Answer from the drawing. Dimensions are ordinates in mm from the lowest x, y and z of the part. Round coordinates to 2 decimals unless told otherwise and drop trailing zeros. Loops run counter-clockwise (first coordinate to the right, second up) from the corner with the lowest first, then second, coordinate; pieces in that order, holes last. Notation, with made-up numbers: M -30.75,-1 L 17.25,-1 A23 ccw 17.25,23 Z; hole C 16.25,21 d9. An arc over 180 degrees is marked long. Answer as a JSON object with one key per item and string values.
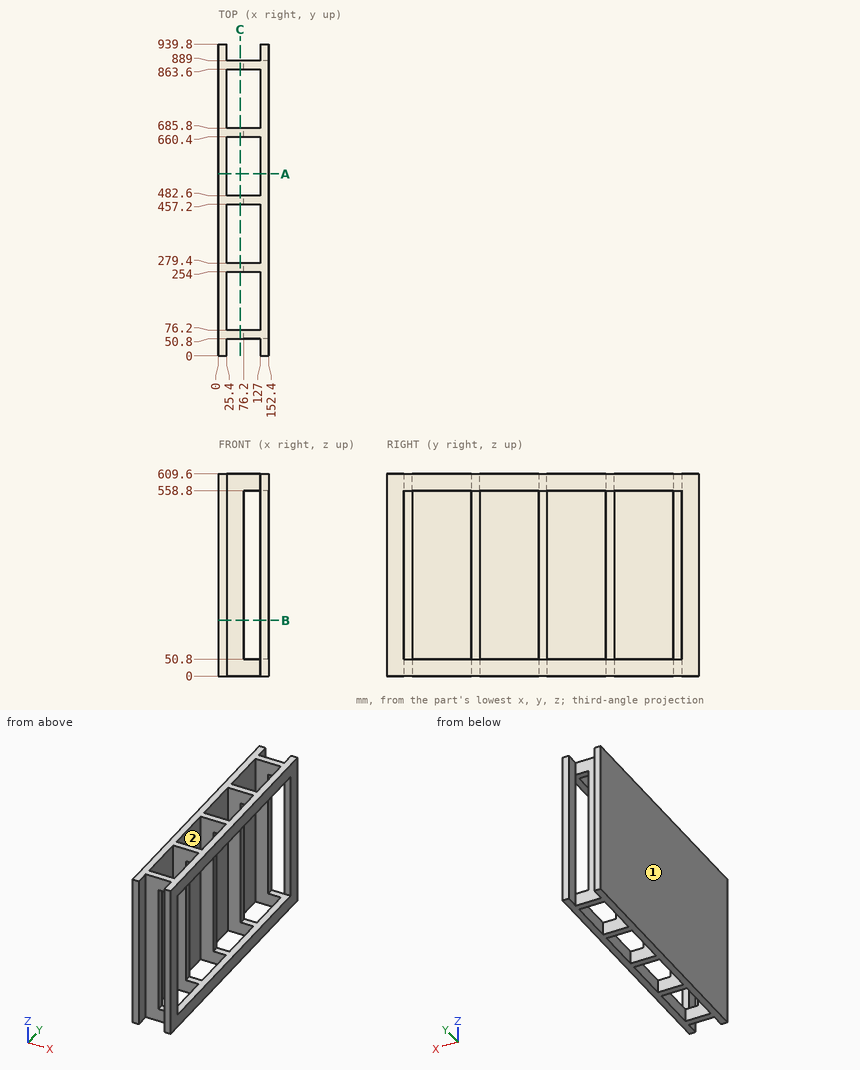
Item 1: The part is cut by section B-B (z = 168). Give the number of separate pieces and of enclosed holes in the cut face, then the cut area to 3 significant figures.
Values follow:
{"separate pieces": "3", "enclosed holes": "0", "area": "32,900 mm^2"}
Item 2: Determine the mould class of the marked faces 1 and 2 for opening direction Y: released by +Y, released by -Y, zero draft, split by the parting line, or undercut.
Values follow:
{"face 1": "zero draft", "face 2": "undercut"}
Item 3: The part is cut by section A-A (y = 548). Give the vertices of the cut face in (x, z).
Values follow:
{"outline": "M 0,0 L 25.4,0 L 25.4,609.6 L 0,609.6 Z; M 127,0 L 152.4,0 L 152.4,50.8 L 127,50.8 Z; M 127,558.8 L 152.4,558.8 L 152.4,609.6 L 127,609.6 Z"}
Item 4: Flat-ended cylindrical pins translate along their axes: P1, Ø5, axis at x = 123.5, y = 701, coming from the -Z side; P2, Ø1.5, axis at y = 220.5, z = 85, coming from the +X side; P3, Ø7.5, axis at y = 266, z = 257, coming from the +X side. Find the tip coordinate at first contact, or state that the pin passes through.
Values follow:
{"P1": "through", "P2": "x = 25.4", "P3": "x = 76.2"}
Item 5: Straight lines are drawn through the part: line 1 (Y direction, x = 76, z = 209); line 2 (Z direction, x = 136.5, y = 631); line 3 (Y direction, x = 138.5, z = 243.5). For each, find the intervals that lie inside material, in ascending order.
Values follow:
{"line 1": "50.8 to 76.2, 254 to 279.4, 457.2 to 482.6, 660.4 to 685.8, 863.6 to 889", "line 2": "0 to 50.8, 558.8 to 609.6", "line 3": "0 to 50.8, 889 to 939.8"}
Item 6: The part is cut by section C-C (x = 65.5). Give the vertices of the cut face in (y, z), then the cut area to 3 significant figures.
Values follow:
{"outline": "M 50.8,0 L 76.2,0 L 76.2,609.6 L 50.8,609.6 Z; M 254,0 L 279.4,0 L 279.4,609.6 L 254,609.6 Z; M 457.2,0 L 482.6,0 L 482.6,609.6 L 457.2,609.6 Z; M 660.4,0 L 685.8,0 L 685.8,609.6 L 660.4,609.6 Z; M 863.6,0 L 889,0 L 889,609.6 L 863.6,609.6 Z", "area": "77,400 mm^2"}
